Build history of the part. All positions in model axes, mm. A direction names the side the tool comes from. Round coordinates to 2 decimals unless told otherwise and drop trailing zeros. Loops run counter-clockwise (first coordinate to the right, second up) from the corner with the lowest first, then second, coordinate; pieces in that order, holes last. Notation, with made-up numbers: M 77,-5 L 89,-5 A25 ccw 89,25 Z; hole C 74,-35 d9. An arc over 180 degrees is marked long. One line per item, written item: value.
```python
from build123d import *

# Parameters (mm, degrees)
SKETCH1_W                     = 46
SKETCH1_H                     = 50
SKETCH1_R                     = 7
BOSS_EXTRUDE1_DEPTH           = 8
FILLET1_R                     = 3
CBORE_FOR_M4_SHCS1_AT_2_COUNT = 2
CBORE_FOR_M4_SHCS1_AT_2_PITCH = 24


with BuildPart() as part:
    # Sketch1 → Boss-Extrude1 (new body)
    with BuildSketch(Plane.XY):
        Rectangle(SKETCH1_W, SKETCH1_H)
        with Locations((0, 12.25)):
            Circle(SKETCH1_R, mode=Mode.SUBTRACT)
    extrude(amount=BOSS_EXTRUDE1_DEPTH)

    # Fillet1
    fillet1_edges = [part.edges().sort_by_distance(p)[0] for p in [
        (23, -25, 4),
        (-23, -25, 4),
        (-23, 25, 4),
        (23, 25, 4),
    ]]
    fillet(fillet1_edges, radius=FILLET1_R)

    # Sketch3 → CBORE for M4 SHCS1 (revolve, cut)
    with BuildSketch(Plane(origin=(-12, -15, 8), x_dir=(0, -1, 0), z_dir=(1, 0, 0))):
        Polygon((0, 0), (0, 8), (2.25, 8), (2.25, 4), (4, 4), (4, 0.025), (4.025, 0), align=None)
    cbore_for_m4_shcs1 = revolve(axis=Axis((-12, -15, 14.35), (0, 0, -1)), mode=Mode.SUBTRACT)

    # CBORE for M4 SHCS1 at 2: CBORE for M4 SHCS1 ×2
    with Locations(*[(i * CBORE_FOR_M4_SHCS1_AT_2_PITCH, 0, 0) for i in range(1, CBORE_FOR_M4_SHCS1_AT_2_COUNT)]):
        add(cbore_for_m4_shcs1, mode=Mode.SUBTRACT)


solid = part.part
```
Item 1: Slice it at D-D, the plane z = 5. Give the cut face in (x, y), and give its area (3 significant figures).
Check values:
outline: M -23,-22 A3 ccw -20,-25 L 20,-25 A3 ccw 23,-22 L 23,22 A3 ccw 20,25 L -20,25 A3 ccw -23,22 Z; hole C -12,-15 d8; hole C 0,12.25 d14; hole C 12,-15 d8
area: 2,040 mm2
Item 2: Slice it at C-C, the plane y = 12.25. Give the cut face in (x, z).
Check values:
outline: M -23,0 L -7,0 L -7,8 L -23,8 Z; M 7,0 L 23,0 L 23,8 L 7,8 Z
Item 3: Pull direction X, two halves, no side cores. Call faces 1 (the face through (-22.14, 24.1, 4.06)), 2 (the face through (0, 25, 4)), 3 (the face through (12, -11, 6)): pulls with the +X half, pulls with the -X half, needs draft (parallel to the pull), parting line crosses it, or undercut.
Check values:
face 1: pulls with the -X half
face 2: needs draft
face 3: undercut
Item 4: Slice it at A-A, the plane x = 12. Give the cut face in (y, z) (3 decimals), and give its area (3 significant figures).
Check values:
outline: M -25,0 L -17.25,0 L -17.25,4 L -19,4 L -19,7.975 L -19.025,8 L -25,8 Z; M -12.75,0 L 25,0 L 25,8 L -10.975,8 L -11,7.975 L -11,4 L -12.75,4 Z
area: 350 mm2
Item 5: Slice it at B-B, the plane y = -15. Give the cut face in (x, z) (3 decimals).
Check values:
outline: M -23,0 L -14.25,0 L -14.25,4 L -16,4 L -16,7.975 L -16.025,8 L -23,8 Z; M -9.75,0 L 9.75,0 L 9.75,4 L 8,4 L 8,7.975 L 7.975,8 L -7.975,8 L -8,7.975 L -8,4 L -9.75,4 Z; M 14.25,0 L 23,0 L 23,8 L 16.025,8 L 16,7.975 L 16,4 L 14.25,4 Z
Item 6: Which spindle directions (+Z, -Z, +X, -X, +Y, -Y) get a long thin tool onto all of the face, cutting with end or side? Do faces 4 (the face through (-10, -13, 4)), 5 (the face through (23, 0, 4)). Say none if no direction does.
Check values:
face 4: +Z
face 5: +Z, -Z, +X, +Y, -Y
Item 7: Drop flat-ended pins along their axis: P1, Ø6, axis at x = -12, y = -15, coming from the +Z side; P2, Ø11, axis at x = 0, y = 12.25, coming from the -Z side. Give the stop position or say it passes through.
Check values:
P1: stops at z = 4
P2: passes through
Item 8: Wall check: line 1 along X through (y, z) = (-15, 7.15); line 2 along X through (y, z) = (-15, 2.2); line 3 along Y through (x, z) = (0, 2.5). Give the ranges that are in metal, low to high.
Check values:
line 1: x = -23 to -16, -8 to 8, 16 to 23
line 2: x = -23 to -14.25, -9.75 to 9.75, 14.25 to 23
line 3: y = -25 to 5.25, 19.25 to 25
